from build123d import *

# Parameters (mm, degrees)
BOSS_EXTRUDE1_DEPTH  = 5
M3_CLEARANCE_HOLE1_D = 3.4
CUT_EXTRUDE1_DEPTH   = 3
CIRPATTERN1_COUNT    = 3
M3_CLEARANCE_HOLE2_D = 3.4


with BuildPart() as part:
    # Sketch1 → Boss-Extrude1 (new body)
    with BuildSketch(Plane.XY):
        with BuildLine():
            Line((0, 17.5), (92.825687176, 17.5))
            ThreePointArc((92.825687176, 17.5), (100.175973433, 0.719639248), (82.858168684, 6.694658386))
            Line((82.858168684, 6.694658386), (17.443157361, 1.409347824))
            ThreePointArc((17.443157361, 1.409347824), (-11.865631317, -12.863000951), (0, 17.5))
        make_face()
    extrude(amount=BOSS_EXTRUDE1_DEPTH)

    # M3 Clearance Hole1 (through all)
    with Locations(Plane.XY.offset(5)):
        with Locations((-12, 0)):
            m3_clearance_hole1 = Hole(M3_CLEARANCE_HOLE1_D / 2)

    # Sketch8 → Cut-Extrude1 (cut)
    with BuildSketch(Plane.XY.offset(5)):
        Polygon((-10.383419246, 2.8), (-13.616580754, 2.8), (-15.233161507, 0), (-13.616580754, -2.8), (-10.383419246, -2.8), (-8.766838493, 0), align=None)
    cut_extrude1 = extrude(amount=-CUT_EXTRUDE1_DEPTH, mode=Mode.SUBTRACT)

    # CirPattern1: M3 Clearance Hole1, Cut-Extrude1 ×3 about axis
    cirpattern1_axis = Axis((0, 0, 0), (0, 0, 1))
    add([m3_clearance_hole1.rotate(cirpattern1_axis, i * 360 / CIRPATTERN1_COUNT) for i in range(1, CIRPATTERN1_COUNT)], mode=Mode.SUBTRACT)
    add([cut_extrude1.rotate(cirpattern1_axis, i * 360 / CIRPATTERN1_COUNT) for i in range(1, CIRPATTERN1_COUNT)], mode=Mode.SUBTRACT)

    # M3 Clearance Hole2 (through all)
    with Locations(Plane.XY.offset(5)):
        with Locations((92.825687176, 7.5)):
            Hole(M3_CLEARANCE_HOLE2_D / 2)


solid = part.part
Part model, mm, in its own coordinate system. A direction names the side the tool comes from. Coordinates: 2 decimals unless noted, no trailing zeros. Order: outer loops, then holes, each group sorted by start corner. A loop starts at its lowest first (then second) coordinate and runs counter-clockwise, first axis right, second up. Notation, with made-up numbers: M -38.5,33.5 L 8.5,33.5 A5 cw 8.5,42.5 Z; hole C 50,54 d2. An arc over 180 degrees is marked long. Use a Markdown table: item, result.
(1) Cut at B-B on x = -12. Write the cut outline in (y, z).
A:
| item | result |
|---|---|
| outline | M -12.74,0 L -1.7,0 L -1.7,2 L -2.8,2 L -2.8,5 L -12.74,5 Z; M 1.7,0 L 12.74,0 L 12.74,5 L 2.8,5 L 2.8,2 L 1.7,2 Z |
(2) Probe L1, parallel to X at y = 1, z = 4.8; L2, parallel to Y at x = 6.5, z = 3.4; L3, parallel to X at y = 8.5, z = 4.05. List the from-to ranges inside material, lowest first.
A:
| item | result |
|---|---|
| L1 | x = -17.47 to -14.66, -9.34 to 17.47, 85.23 to 100.43 |
| L2 | y = -16.25 to -13.19, -7.59 to 7.59, 13.19 to 17.5 |
| L3 | x = -15.3 to 3.86, 8.14 to 91.45, 94.2 to 102.78 |
(3) Flat gauge pins, fed straight in: pin 1 (1.5 mm diameter, centred on x = 39.5, z = 2, fed in from -Y); pin 2 (2 mm diameter, centred on x = 92.83, y = 7.5, fed in from -Z); pin 3 (2.5 mm diameter, centred on x = 6, z = 4, fed in from -Y); pin 4 (1 mm diameter, centred on y = -0.5, z = 3, fed in from +X). Where does each tip first touch, or does it go through?
A:
| item | result |
|---|---|
| pin 1 | stops at y = 3.13 |
| pin 2 | passes through |
| pin 3 | stops at y = -16.84 |
| pin 4 | stops at x = 99.44 |
(4) Cut at D-D on x = 62. Write the cut outline in (y, z).
A:
| item | result |
|---|---|
| outline | M 5.01,0 L 17.5,0 L 17.5,5 L 5.01,5 Z |
(5) Pull direction X, two halves, no side cores. Call faces 3 (the flat face through (30, 8, 5)), 4 (the flat face through (6, -7.592, 4)), 5 (the cylindrical face through (6.37, -12.05, 0.99)): released by +X, released by -X, zero draft, split by the parting line, or undercut.
A:
| item | result |
|---|---|
| face 3 | zero draft |
| face 4 | undercut |
| face 5 | undercut |
(6) Tool access for faces 1 (the cylindrical face through (6.369, 8.733, 0.986)), 2 (the flat face through (6, 7.592, 4)): list every direction of +Z, -Z, +X, -X, +Y, -Y with a clear straight run to the whole face (end or side of a thin tool).
A:
| item | result |
|---|---|
| face 1 | +Z, -Z |
| face 2 | +Z |
(7) Cut at A-A on z = 3.3. Write the cut outline in (x, y), then the cut area to 3 significant figures.
A:
| item | result |
|---|---|
| outline | M 0,17.5 A17.5 ccw long 17.44,1.41 L 82.86,6.69 A10 ccw long 92.83,17.5 Z; hole M -15.23,0 L -13.62,-2.8 L -10.38,-2.8 L -8.77,0 L -10.38,2.8 L -13.62,2.8 Z; hole M 2.77,-10.39 L 4.38,-13.19 L 7.62,-13.19 L 9.23,-10.39 L 7.62,-7.59 L 4.38,-7.59 Z; hole M 2.77,10.39 L 4.38,7.59 L 7.62,7.59 L 9.23,10.39 L 7.62,13.19 L 4.38,13.19 Z; hole C 92.83,7.5 d3.4 |
| area | 2,150 mm^2 |
(8) Cut at C-C on y = -4.5. Write the cut outline in (x, z), then the cut area to 3 significant figures.
A:
| item | result |
|---|---|
| outline | M -16.91,0 L 16.91,0 L 16.91,5 L -16.91,5 Z |
| area | 169 mm^2 |
